from build123d import *

# Parameters (mm, degrees)
F1_DEPTH = 170.6
F2_R     = 5.0100682876
F3_DEPTH = 12.3
F5_DEPTH = 19
F5_TAPER = 12


with BuildPart() as f1:
    # F0 (on Top) → F1 (new body)
    with BuildSketch(Plane.XY):
        Polygon((-15.8018649923, 17.5146961328), (-12.1233743963, 20.9012440706), (-13.2169656436, 25.7801843433), (-17.9890474869, 27.2725766781), (-21.6675380829, 23.8860287403), (-20.5739468356, 19.0070884677), align=None)
    extrude(amount=F1_DEPTH)

    # F2 (on face) → F3 (join)
    with BuildSketch(Plane(origin=(0, 0, 0), x_dir=(1, 0, 0), z_dir=(0, 0, -1))):
        with Locations((-16.9993620366, -22.4947221577)):
            Circle(F2_R)
    extrude(amount=F3_DEPTH)

    # F4 (on face) → F5 (join)
    with BuildSketch(Plane.XY.offset(170.6)):
        with BuildLine():
            ThreePointArc((-13.7097899359, 25.3264729507), (-19.8282927849, 25.5793027092), (-20.0811225433, 19.4607998602))
            Line((-20.0811225433, 19.4607998602), (-13.7097899359, 25.3264729507))
        make_face()
        with BuildLine():
            Line((-13.7097899359, 25.3264729507), (-20.0811225433, 19.4607998602))
            ThreePointArc((-20.0811225433, 19.4607998602), (-15.3213437492, 18.3597586349), (-12.5653292207, 22.3936364055))
            ThreePointArc((-12.5653292207, 22.3936364055), (-12.8615784691, 23.9677488959), (-13.7097899359, 25.3264729507))
        make_face()
    extrude(amount=F5_DEPTH, taper=F5_TAPER)


solid = f1.part
Here's how the part is built. I have some questions about the finished solid (model axes, mm). A direction names the side the tool comes from. Give positions to 0.01 mm unless a question says otherwise; leave off trailing zeros. Order: outer loops, then holes, each group sorted by start corner. A loop starts at its lowest first (then second) coordinate and runs counter-clockwise, first axis right, second up. Notation, with made-up numbers: M 74.5,-25.5 L 106.5,-25.5 A4 ccw 106.5,-18.5 Z; hole C 78,69 d9. An arc over 180 degrees is marked long. Answer as a JSON object with one key per item and string values. Group by question number.
1) On a 3-axis mill with a long thin cutter (end or side, diameter ignored), from which of +Z, -Z, +X, -X, +Y, -Y can I reach the whole of each face in a straight line? I mean faces 1 (the flat face through (-18.22, 18.27, 84.11)), 2 (the flat face through (-13.988, 19.184, 84.106)), 3 (the flat face through (-21, 25, 0)), 4 (the flat face through (-12.663, 23.307, 84.106)). Say none if no direction works.
2) Please list where these lines run through material, in increasing order: L1, parallel to Z at x = -21, y = 20.5; L2, parallel to X at y = 24.5, z = 113.5; L3, parallel to X at y = 22.75, z = 5.5. Write a range as [from, to].
3) Suppose I cut it at A-A, the plane z = 84.5. Write out the boundary of the cut face in (x, y).
4) I'm going to push flat-ended pins straight in: pin 1 Ø2 at (x, z) = (-14.5, 109) entering from -Y; pin 2 Ø3 at (x, z) = (-16.5, 141.5) entering from -Y; pin 3 Ø1.5 at (x, z) = (-15, 78) entering from +Y. Where does each tip first touch, or does it pass through?
Results found:
{
 "1": {"face 1": "+Z, -X, -Y", "face 2": "+Z, +X, -Y", "face 3": "+Z", "face 4": "+Z, +X, +Y"},
 "2": {"L1": "[-12.3, 0]", "L2": "[-21, -12.93]", "L3": "[-21.41, -12.54]"},
 "3": {"outline": "M -21.67,23.89 L -20.57,19.01 L -15.8,17.51 L -12.12,20.9 L -13.22,25.78 L -17.99,27.27 Z"},
 "4": {"pin 1": "y = 17.79", "pin 2": "y = 17.51", "pin 3": "y = 26.57"}
}
